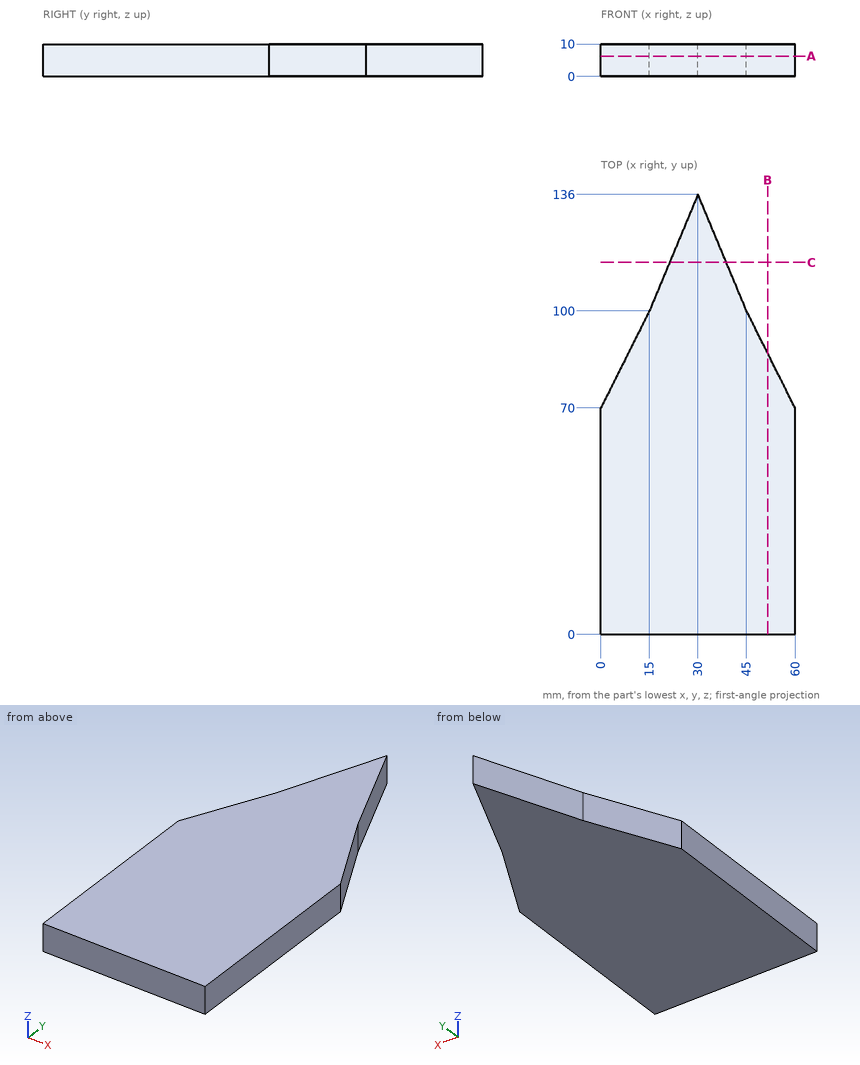
Here's the drawing with two shaded views (mm, measured from the low corner). I have some questions. Give positions to 0.01 mm unless a question says otherwise; leave off trailing zeros. Loops run counter-clockwise (first coordinate to the right, second up) from the corner with the lowest first, then second, coordinate; pieces in that order, holes last. Notation, with made-up numbers: (-9.75, 37.25) -> (34.25, 37.25) arc R16 cw to (34.25, 51.25) -> close; hole circle Ø7 at (54.5, 17.25). An arc over 180 degrees is marked (long way). Use one line per item in the form item = value.
1) Will these pins go through, and if not, where does the flat tip stop? pin 1 (6 mm diameter, centred on x = 19, z = 8.5, fed in from +Y); pin 2 (6 mm diameter, centred on x = 53, z = 6, fed in from +Y); pin 3 (3 mm diameter, centred on x = 16, z = 6, fed in from +Y).
Answers:
pin_1 = 116.8
pin_2 = 90
pin_3 = 106
2) If we section it at C-C (y = 115): Please give me the cut outline in (x, z).
Answers:
outline = (21.25, 0) -> (38.75, 0) -> (38.75, 10) -> (21.25, 10) -> close
3) If we section it at B-B (x = 51.5): Please give me the cut outline in (y, z), plus the area to 3 significant figures.
Answers:
outline = (0, 0) -> (87, 0) -> (87, 10) -> (0, 10) -> close
area = 870 mm²
4) If we section it at A-A (z = 6.25): Please give me the cut outline in (x, y).
Answers:
outline = (0, 0) -> (60, 0) -> (60, 70) -> (45, 100) -> (30, 136) -> (15, 100) -> (0, 70) -> close
5) I need wall thicknesses on line 1 along Y through (x, z) = (15, 4); line 2 along X through (y, z) = (86, 7.5); line 3 along Y through (x, z) = (23.5, 5.25). Which ranges of each line are inside material? Lowest first, please.
Answers:
line_1 = 0 to 100
line_2 = 8 to 52
line_3 = 0 to 120.4
